from build123d import *

# Parameters (mm, degrees)
SKETCH_1_W          = 60
SKETCH_1_H          = 40
EXTRUDE_1_DEPTH     = 5
SKETCH_3_W          = 60
SKETCH_3_H          = 5
EXTRUDE_2_DEPTH     = 25
SKETCH_4_W          = 60
SKETCH_4_H          = 5
EXTRUDE_3_DEPTH     = 10
SKETCH_5_R          = 1.5
CUT_EXTRUDE_1_DEPTH = 5


with BuildPart() as part:
    # Эскиз1 → Бобышка-Вытянуть1 (new body)
    with BuildSketch(Plane(origin=(0, 0, 0), x_dir=(1, 0, 0), z_dir=(0, 1, 0))):
        Rectangle(SKETCH_1_W, SKETCH_1_H)
    extrude(amount=EXTRUDE_1_DEPTH)

    # Эскиз3 → Бобышка-Вытянуть2 (add)
    with BuildSketch(Plane(origin=(0, 5, 0), x_dir=(1, 0, 0), z_dir=(0, 1, 0))):
        with Locations((0, 17.5)):
            Rectangle(SKETCH_3_W, SKETCH_3_H)
    extrude(amount=EXTRUDE_2_DEPTH)

    # Эскиз4 → Бобышка-Вытянуть3 (add)
    with BuildSketch(Plane.XY.offset(-15)):
        with Locations((0, 27.5)):
            Rectangle(SKETCH_4_W, SKETCH_4_H)
    extrude(amount=EXTRUDE_3_DEPTH)

    # Эскиз5 → Вырез-Вытянуть1 (cut)
    with BuildSketch(Plane.XZ):
        with Locations(Location((22, -10, 0), (0, 0, 270))):
            Circle(SKETCH_5_R)
        with Locations(Location((-22, -10, 0), (0, 0, 270))):
            Circle(SKETCH_5_R)
    extrude(amount=-CUT_EXTRUDE_1_DEPTH, mode=Mode.SUBTRACT)


solid = part.part
The listing builds one solid part. Answer for the finished solid, in the listing's coordinates (mm). A direction names the side the tool comes from. Coordinates: 2 decimals unless noted, no trailing zeros. Write each loop counter-clockwise with the first axis right and the second up, starting at its lowest first coordinate (ties: lowest second). Pieces come first, ordered by that corner, then holes. Notation, with made-up numbers: M 23.5,53 L 54.5,53 A35 ccw 54.5,90 Z; hole C 31,56 d10. An arc over 180 degrees is marked long. Write each question's results on one line, items separated by ' | '.
Item 1: The part is cut by section D-D on y = 24. Determine the outline of the cut face in (x, z).
Answer below:
outline: M -30,-20 L 30,-20 L 30,-15 L -30,-15 Z
Item 2: The part is cut by section C-C on x = -5.5. Determine the outline of the cut face in (y, z), and give its area (3 significant figures).
Answer below:
outline: M 0,-20 L 30,-20 L 30,-5 L 25,-5 L 25,-15 L 5,-15 L 5,20 L 0,20 Z | area: 375 mm2
Item 3: Given P1, Ø3, axis at y = 18.5, z = -13, coming from the +X side; P2, Ø2.5, axis at x = -10.5, y = 26.5, coming from the +Z side; P3, Ø1.5, axis at x = 7, y = 20.5, coming from the +Z side, each flat-ended and moving along its own axis, determine where each tip first touches the part or whether it passes through.
Answer below:
P1: through | P2: z = -5 | P3: z = -15
Item 4: The part is cut by section A-A on x = 22. Determine the outline of the cut face in (y, z).
Answer below:
outline: M 0,-20 L 30,-20 L 30,-5 L 25,-5 L 25,-15 L 5,-15 L 5,-11.5 L 0,-11.5 Z; M 0,-8.5 L 5,-8.5 L 5,20 L 0,20 Z
Item 5: The part is cut by section B-B on z = -10. Determine the outline of the cut face in (x, y).
Answer below:
outline: M -30,0 L -23.5,0 L -23.5,5 L -30,5 Z; M -30,25 L 30,25 L 30,30 L -30,30 Z; M -20.5,0 L 20.5,0 L 20.5,5 L -20.5,5 Z; M 23.5,0 L 30,0 L 30,5 L 23.5,5 Z
Item 6: Which of the six approach directions +Z, -Z, +X, -X, +Y, -Y give full straight-line access (tool end or side, diameter ignored) to faces 5 (the face through (0, 5, 2)), 6 (the face through (0, 28, -5)), 7 (the face through (23.487, 2.465, -9.805)), 8 (the face through (30, 4, -8))?
Answer below:
face 5: +Z, +X, -X | face 6: +Z, +X, -X, +Y | face 7: -Y | face 8: +Z, -Z, +X, +Y, -Y
Item 7: For a pull along Y with two mould halves and no side action, classify faces 1 (the face through (0, 0, 0)), 2 (the face through (0, 15, -20)), 3 (the face through (0, 15, -15)), 4 (the face through (0, 30, -13)) as released by +Y, released by -Y, zero draft, split by the parting line, or undercut.
Answer below:
face 1: released by -Y | face 2: zero draft | face 3: undercut | face 4: released by +Y
Item 8: Consider probe 1 along X at (y, z) = (2.2, -10); probe 2 along Y at (x, z) = (-15, -14.5); probe 3 along Y at (x, z) = (-25.5, 17.5). Determine where each line is inside the solid, lowest interval first. Write a range as [from, to].
Answer below:
probe 1: [-30, -23.5], [-20.5, 20.5], [23.5, 30] | probe 2: [0, 5], [25, 30] | probe 3: [0, 5]
